Autodesk Inventor part; units mm, degrees
ref_plane "YZ Plane" through (0, 0, 0) normal (1, 0, 0) x (0, 1, 0)
ref_plane "XZ Plane" through (0, 0, 0) normal (0, 1, 0) x (-1, 0, 0)
ref_plane "XY Plane" through (0, 0, 0) normal (0, 0, 1) x (1, 0, 0)
sketch "Sketch1" plane through (0, 0, 0) normal (0, 1, 0) x (-1, 0, 0)
  line L0 (-0.5, 18.5) -> (-12.5, 18.5)
  line L1 (-12.5, 18.5) -> (-12.5, -18.5)
  line L2 (-12.5, -18.5) -> (-0.5, -18.5)
  line L3 (-0.5, -18.5) -> (-0.5, 18.5)
  line L4 (12.5, 18.5) -> (0.5, 18.5)
  line L5 (0.5, 18.5) -> (0.5, -18.5)
  line L6 (0.5, -18.5) -> (12.5, -18.5)
  line L7 (12.5, -18.5) -> (12.5, 18.5)
  line L8 (15.5, 18.5) -> (-15.5, 18.5)
  line L9 (-15.5, 18.5) -> (-15.5, -18.5)
  line L10 (-15.5, -18.5) -> (15.5, -18.5)
  line L11 (15.5, -18.5) -> (15.5, 18.5)
  point P0 (0, 0)
  point P1 (-12.5, -18.5)
  point P2 (-12.5, 18.5)
  point P3 (-0.5, -18.5)
  point P4 (0.5, -18.5)
  point P5 (0.5, 18.5)
  point P6 (-0.5, 18.5)
  point P7 (12.5, 18.5)
  point P8 (12.5, -18.5)
  dimension "d0" = 12
  dimension "d1" = 12
  dimension "d2" = 1
  dimension "d3" = 37
  dimension "d4" = 37
  dimension "d5" = 0
  dimension "d6" = 0.5
  dimension "d7" = 18.5
  dimension "d8" = 3
  dimension "d9" = 3
  dimension "d10" = 0
  dimension "d11" = 0
extrude "Extrusion1" add sketch "Sketch1" along normal blind 15.5 contours L8 L5 L10 L3 | L1 L10 L9 L8 | L8 L11 L10 L7
sketch "Sketch2" plane through (0, 0, 0) normal (0, -1, 0) x (1, 0, 0)
  line L0 (24.5, 28) -> (-24.5, 28)
  line L1 (-24.5, 28) -> (-24.5, -28)
  line L2 (-24.5, -28) -> (24.5, -28)
  line L3 (24.5, -28) -> (24.5, 28)
  line L4 (15.5, 18.5) -> (15.5, -18.5)
  line L5 (-15.5, -18.5) -> (-15.5, 18.5)
  line L6 (24.5, 28) -> (-24.5, 28)
  line L7 (-24.5, 28) -> (-24.5, 31)
  line L8 (-24.5, 31) -> (24.5, 31)
  line L9 (24.5, 31) -> (24.5, 28)
  line L10 (-24.5, -28) -> (24.5, -28)
  line L11 (24.5, -28) -> (24.5, -31)
  line L12 (24.5, -31) -> (-24.5, -31)
  line L13 (-24.5, -31) -> (-24.5, -28)
  point P0 (0, 0)
  point P1 (24.5, -28)
  point P2 (-24.5, 28)
  dimension "d14" = 56
  dimension "d15" = 28
  dimension "d16" = 9
  dimension "d17" = 9
  dimension "d18" = 3
  dimension "d19" = 3
extrude "Extrusion2" add sketch "Sketch2" along normal blind 3
sketch "Sketch3" plane through (0, -3, 0) normal (0, -1, 0) x (1, 0, 0)
  line L0 (24.5, 28) -> (-24.5, 28)
  line L1 (-24.5, 28) -> (-24.5, -28)
  line L2 (-24.5, -28) -> (24.5, -28)
  line L3 (24.5, -28) -> (24.5, 28)
  line L4 (24.5, 28) -> (-24.5, 28)
  line L5 (-24.5, 28) -> (-24.5, 31)
  line L6 (-24.5, 31) -> (24.5, 31)
  line L7 (24.5, 31) -> (24.5, 28)
  line L8 (-24.5, -28) -> (24.5, -28)
  line L9 (24.5, -28) -> (24.5, -31)
  line L10 (24.5, -31) -> (-24.5, -31)
  line L11 (-24.5, -31) -> (-24.5, -28)
  point P0 (0, 0)
  point P1 (24.5, -28)
  point P2 (-24.5, 28)
  point P3 (-24.5, 28)
  point P4 (24.5, -28)
  dimension "d22" = 56
  dimension "d23" = 28
  dimension "d26" = 3
  dimension "d27" = 3
extrude "Extrusion3" add sketch "Sketch3" along normal blind 35 contours L0 L5 L6 L7 | L9 L10 L11 L2
sketch "Sketch4" plane through (0, -38, 0) normal (0, -1, 0) x (1, 0, 0)
  line L0 (24.5, 28) -> (-24.5, 28)
  line L1 (-24.5, 28) -> (-24.5, -28)
  line L2 (-24.5, -28) -> (24.5, -28)
  line L3 (24.5, -28) -> (24.5, 28)
  line L4 (24.5, 28) -> (-24.5, 28)
  line L5 (-24.5, 28) -> (-24.5, 31)
  line L6 (-24.5, 31) -> (24.5, 31)
  line L7 (24.5, 31) -> (24.5, 28)
  line L8 (-24.5, -28) -> (24.5, -28)
  line L9 (24.5, -28) -> (24.5, -31)
  line L10 (24.5, -31) -> (-24.5, -31)
  line L11 (-24.5, -31) -> (-24.5, -28)
  point P0 (0, 0)
  point P1 (24.5, -28)
  point P2 (-24.5, 28)
  dimension "d30" = 56
  dimension "d31" = 28
  dimension "d34" = 3
  dimension "d35" = 3
extrude "Extrusion4" add sketch "Sketch4" along normal blind 3
sketch "Sketch7" plane through (0, -41, 0) normal (0, -1, 0) x (1, 0, 0)
  circle A0 centre (0, 0) radius 6.5
  dimension "d45" = 13
extrude "Extrusion7" add sketch "Sketch7" against normal blind 6
sketch "Sketch8" plane through (0, -41, 0) normal (0, -1, 0) x (1, 0, 0)
  circle A0 centre (0, 0) radius 3.75
  circle A1 centre (0, 0) radius 5
  dimension "d48" = 7.5
  dimension "d49" = 10
extrude "Extrusion8" cut sketch "Sketch8" against normal blind 5
sketch "Sketch9" plane through (0, -41, 0) normal (0, -1, 0) x (1, 0, 0)
  circle A0 centre (0, 0) radius 3.75
  circle A1 centre (0, 0) radius 5
  circle A2 centre (0, 0) radius 6.5
  dimension "d52" = 13
  dimension "d53" = 10
  dimension "d54" = 7.5
extrude "Extrusion9" add sketch "Sketch9" along normal blind 5
properties part number "Koszyk"
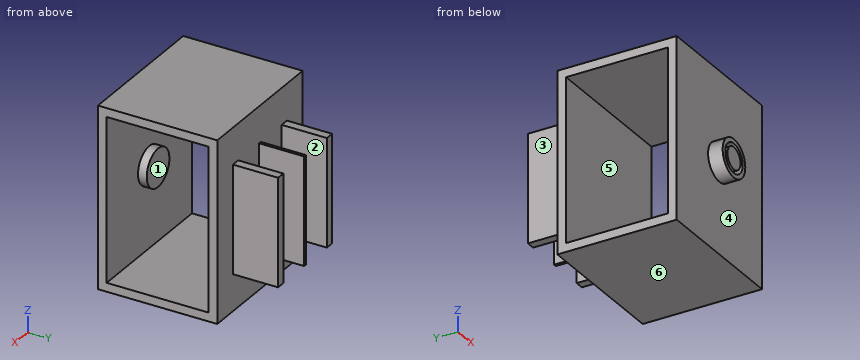
CAD build for the part. Positions are in the model's coordinates, mm. Face numbers are marked on the shaded views. A direction names the side the tool comes from. Give positions to 0.01 mm unless a question says otherwise; leave off trailing zeros. Loops run counter-clockwise (first coordinate to the right, second up) from the corner with the lowest first, then second, coordinate; pieces in that order, holes last. Notation, with made-up numbers: M 9.25,53 L 15.25,53 A27 ccw 15.25,75 Z; hole C 14.25,68 d5. An arc over 180 degrees is marked long. One line per question, with ' | ' between items. Start each with the question number.
1. 3-axis set-ups, long thin cutter, end or side, ignore diameter. For the marked faces 1, 2 and 3: which of +Z, -Z, +X, -X, +Y, -Y reach the whole face in a straight line?
2. Saw through at B-B on y = 1.5. Give the cut face in (x, z), plus the area to 3 significant figures.
3. Two-plate mould, pull along Y, no slides. Class the marked faces 4, 5 and 6: pulls with the +Y half, pulls with the -Y half, needs draft (parallel to the pull), parting line crosses it, or undercut.
4. Flat gauge pins, fed straight in: pin 1 (1.5 mm diameter, centred on x = 14.5, y = 9, fed in from -Z); pin 2 (12 mm diameter, centred on x = -9, z = -9.5, fed in from -Y); pin 3 (3.5 mm diameter, centred on x = 13.5, y = 5.5, fed in from +Z). Where does each tip first touch, or does it go through?
5. Saw through at C-C on y = -24. Give the cut face in (x, z), plus the area to 3 significant figures.
6. Saw through at A-A on z = 9.5. Give the cut face in (x, y), plus the area to 4 significant figures.
7. Saw through at D-D on z = -25.5. Give the cut face in (x, y), plus the area to 3 significant figures.
8. Probe L1, parallel to Z at x = 0, y = -43; L2, parallel to Z at x = 0, y = -38.25; L3, parallel to X at y = 7.5, z = -9. List the from-to ranges inside material, lowest first. Write a range as from..to.
Result sheet:
1) face 1: +X, -X | face 2: +Z, -Z, +Y | face 3: +Z, -Z, -X, +Y
2) outline: M -15.5,-18.5 L -12.5,-18.5 L -12.5,18.5 L -15.5,18.5 Z; M -0.5,-18.5 L 0.5,-18.5 L 0.5,18.5 L -0.5,18.5 Z; M 12.5,-18.5 L 15.5,-18.5 L 15.5,18.5 L 12.5,18.5 Z | area: 259 mm^2
3) face 4: pulls with the -Y half | face 5: undercut | face 6: needs draft
4) pin 1: stops at z = -18.5 | pin 2: stops at y = -41 | pin 3: stops at z = 18.5
5) outline: M -24.5,-31 L 24.5,-31 L 24.5,-28 L -24.5,-28 Z; M -24.5,28 L 24.5,28 L 24.5,31 L -24.5,31 Z | area: 294 mm^2
6) outline: M -24.5,-41 L 24.5,-41 L 24.5,-38 L -24.5,-38 Z; M -24.5,-3 L 24.5,-3 L 24.5,0 L 15.5,0 L 15.5,15.5 L 12.5,15.5 L 12.5,0 L 0.5,0 L 0.5,15.5 L -0.5,15.5 L -0.5,0 L -12.5,0 L -12.5,15.5 L -15.5,15.5 L -15.5,0 L -24.5,0 Z | area: 402.5 mm^2
7) outline: M -24.5,-41 L 24.5,-41 L 24.5,-38 L -24.5,-38 Z; M -24.5,-3 L 24.5,-3 L 24.5,0 L -24.5,0 Z | area: 294 mm^2
8) L1: z = -6.5..-5, -3.75..3.75, 5..6.5 | L2: z = -31..-5, -3.75..3.75, 5..31 | L3: x = -15.5..-12.5, -0.5..0.5, 12.5..15.5
